Autodesk Inventor part; units mm, degrees
ref_plane "YZ Plane" through (0, 0, 0) normal (1, 0, 0) x (0, 1, 0)
ref_plane "XZ Plane" through (0, 0, 0) normal (0, 1, 0) x (-1, 0, 0)
ref_plane "XY Plane" through (0, 0, 0) normal (0, 0, 1) x (1, 0, 0)
sketch "Sketch1" plane through (0, 0, 0) normal (1, 0, 0) x (0, 1, 0)
  line L0 (0, 0) -> (0, -15.9233)
  line L1 (0, -15.9233) -> (3.236, -15.9233)
  line L2 (3.236, -15.9233) -> (3.236, -24.1071)
  line L3 (3.236, -24.1071) -> (6.4618, -24.1071)
  line L4 (6.4618, -24.1071) -> (6.4618, -32.2859)
  line L5 (6.4618, -32.2859) -> (9.6876, -32.2859)
  line L6 (0, 0) -> (2.2149, 0)
  line L7 (9.6876, -32.2859) -> (40.3351, -32.2859) construction
  arc A0 (9.6876, -32.2859) -> (2.2149, 0) centre (-65.2438, -32.6213) ccw
  dimension "d0" = 15.9233
  dimension "d1" = 3.236
  dimension "d2" = 3.2258
  dimension "d3" = 3.2258
  dimension "d4" = 24.1071
  dimension "d5" = 32.2859
  dimension "d6" = 2.2149
extrude "Extrusion1" add sketch "Sketch1" along normal blind 7.7978
shell "Shell1" thickness 1.4732 removed faces 3 at (2.5993, 0, -5.3078) at (2.5993, 3.236, -18.6512) at (2.5993, 6.4618, -26.8334)
sketch "Sketch5" plane through (0, 3.236, -24.1071) normal (0, -1, 0) x (1, 0, 0)
  line L0 (6.3246, 8.1839) -> (7.7978, 8.1839)
  line L1 (7.7978, 8.1839) -> (1.4732, 8.1839)
  line L2 (1.4732, 8.1839) -> (1.4732, 9.6571)
  line L3 (1.4732, 9.6571) -> (7.7978, 9.6571)
  line L4 (7.7978, 9.6571) -> (7.7978, 8.1839)
  line L5 (0, 8.1839) -> (1.4732, 8.1839)
  line L6 (1.4732, 9.6571) -> (0, 9.6571)
  line L7 (0, 9.6571) -> (0, 8.1839)
  line L8 (0, 8.1839) -> (1.4732, 8.1839)
  line L9 (1.4732, 8.1839) -> (1.4732, 9.6571)
  point P0 (0, 24.1071)
extrude "Extrusion2" add sketch "Sketch5" against normal up to surface
sketch "Sketch8" plane through (0, 3.236, -24.1071) normal (0, -1, 0) x (1, 0, 0)
  line L0 (1.4732, 1.4732) -> (6.3246, 1.4732)
  line L1 (6.3246, 1.4732) -> (1.4732, 1.4732)
  line L2 (1.4732, 1.4732) -> (1.4732, 0)
  line L3 (1.4732, 0) -> (6.3246, 0)
  line L4 (6.3246, 0) -> (6.3246, 1.4732)
  point P0 (0, 24.1071)
  point P1 (7.7978, 0)
  point P2 (0, 0)
extrude "Extrusion3" add sketch "Sketch8" against normal up to surface
sketch "Sketch9" plane through (0, 0, -15.9233) normal (0, -1, 0) x (1, 0, 0)
  line L0 (1.4732, -6.7107) -> (1.4732, 0)
  line L1 (6.3246, 1.4732) -> (1.4732, 1.4732)
  line L2 (1.4732, 1.4732) -> (1.4732, 14.4501)
  line L3 (1.4732, 14.4501) -> (6.3246, 14.4501)
  line L4 (6.3246, 14.4501) -> (6.3246, 1.4732)
  line L5 (0, 15.9233) -> (0, 0)
  line L6 (0, 0) -> (7.7978, 0)
  line L7 (7.7978, 15.9233) -> (7.7978, 0)
  line L8 (0, 15.9233) -> (7.7978, 15.9233)
  line L9 (0, -8.1839) -> (7.7978, -8.1839)
  line L10 (7.7978, 0) -> (7.7978, -8.1839)
  line L11 (6.3246, 0) -> (7.7978, 0)
  line L12 (6.3246, 0) -> (6.3246, -6.7107)
  line L13 (6.3246, -6.7107) -> (1.4732, -6.7107)
  line L14 (1.4732, -6.7107) -> (1.4732, 0)
  line L15 (0, 0) -> (1.4732, 0)
  line L16 (0, 0) -> (0, -8.1839)
  line L17 (1.4732, -14.8895) -> (1.4732, -8.1839)
  line L18 (0, -8.1839) -> (1.4732, -8.1839)
  line L19 (0, -8.1839) -> (0, -16.3627)
  line L20 (0, -16.3627) -> (7.7978, -16.3627)
  line L21 (7.7978, -8.1839) -> (7.7978, -16.3627)
  line L22 (6.3246, -8.1839) -> (7.7978, -8.1839)
  line L23 (6.3246, -8.1839) -> (6.3246, -14.8895)
  line L24 (6.3246, -14.8895) -> (1.4732, -14.8895)
  line L25 (6.3246, 0) -> (1.4732, 0)
  line L26 (6.3246, -6.7107) -> (1.4732, -6.7107)
  line L27 (4.5491, -1.7297) -> (3.2487, -1.7297)
  line L28 (3.2487, 0) -> (3.2487, -1.7297)
  line L29 (4.5491, -1.7297) -> (4.5491, 0)
  line L30 (4.5491, 0) -> (3.2487, 0)
extrude "Extrusion4" add sketch "Sketch9" against normal up to next from surface at -3.236 contours L6 L29 L27 L28
properties part number "3x1 curve" material "ABS Plastic"
Geometry check sheet. Reference: the model listing, model coordinates, mm. A direction names the side the tool comes from. Round coordinates to 2 decimals unless told otherwise and drop trailing zeros. Write each loop counter-clockwise with the first axis right and the second up, starting at its lowest first coordinate (ties: lowest second). Pieces come first, ordered by that corner, then holes. Notation, with made-up numbers: (51.25, 64.5) - (75.25, 64.5) arc R19 ccw to (75.25, 78.5) - close; hole circle Ø10 at (54.5, 53). An arc over 180 degrees is marked (long way). One line per item, written item: value.
1. Depth check by flat-ended pin: pin 1 Ø3.5 at (x, y) = (3, 1.5) entering from +Z; pin 2 Ø2 at (x, y) = (5, 5) entering from +Z; pin 3 Ø1.5 at (x, z) = (6, -24.5) entering from +Y; pin 4 Ø3.5 at (x, y) = (3.5, 4.5) entering from +Z. Enter the tip coordinate at first touch or a pass-through.
The answers:
pin 1: stops at z = 0
pin 2: stops at z = -3.98
pin 3: stops at y = 9.32
pin 4: stops at z = -1.13
2. Cross-section at D-D on z = -13.5. Record the boundary of the cut face in (x, y).
The answers:
outline: (0, 0) - (1.47, 0) - (1.47, 5.68) - (6.32, 5.68) - (6.32, 0) - (7.8, 0) - (7.8, 7.21) - (0, 7.21) - close
3. Scan lines: L1, parallel to X at y = 0.5, z = -2.5; L2, parallel to Z at x = 4, y = 1.25; L3, parallel to Z at x = 5, y = 2.75. Record each from-to range of solid material in increasing order.
The answers:
L1: x = 0 to 1.47, 6.32 to 7.8
L2: z = -15.92 to -14.45, -1.47 to 0
L3: z = -15.92 to -14.45, -4.82 to -1.13
4. Set-up check for faces 5 (the face through (4, 3.236, -23)), 6 (the face through (4, 8, -27)), 7 (the face through (3.844, 7.705, -15.497)): record each of +Z, -Z, +X, -X, +Y, -Y from which the full face is reachable in a straight line by a thin tool's end or side.
The answers:
face 5: -Z, +X, -X, -Y
face 6: -Y
face 7: +Z, +X, -X, +Y
5. Mould release check, pull along Z, two halves, no side actions. Record for faces 1 (the face through (4, 1, 0)), 2 (the face through (4, 7, -30.813)), 3 (the face through (4, 8, -32.286)), 4 (the face through (1, 0, -8)): released by +Z, released by -Z, zero draft, split by the parting line, or undercut.
The answers:
face 1: released by +Z
face 2: undercut
face 3: released by -Z
face 4: zero draft
6. Cross-section at B-B on y = 1. Record the boundary of the cut face in (x, z), and give its area (3 significant figures).
The answers:
outline: (0, -15.92) - (7.8, -15.92) - (7.8, 0) - (0, 0) - close; hole (1.47, -14.45) - (6.32, -14.45) - (6.32, -1.47) - (1.47, -1.47) - close
area: 61.2 mm^2
7. Cross-section at C-C on y = 4.25. Record the boundary of the cut face in (x, z).
The answers:
outline: (0, -24.11) - (7.8, -24.11) - (7.8, -4.6) - (0, -4.6) - close; hole (1.47, -22.63) - (6.32, -22.63) - (6.32, -15.92) - (4.55, -15.92) - (4.55, -17.65) - (3.25, -17.65) - (3.25, -15.92) - (1.47, -15.92) - close; hole (1.47, -14.45) - (6.32, -14.45) - (6.32, -8.81) - (1.47, -8.81) - close
8. Cross-section at A-A on x = 0.75. Record the boundary of the cut face in (y, z), and give its area (3 significant figures).
The answers:
outline: (0, -15.92) - (3.24, -15.92) - (3.24, -24.11) - (6.46, -24.11) - (6.46, -32.29) - (9.69, -32.29) arc R74.93 ccw to (2.21, 0) - (0, 0) - close
area: 154 mm^2
